```python
from build123d import *

# Parameters (mm, degrees)
ESBO_O1_W                = 12.7
ESBO_O1_H                = 41.5
ESBO_O1_R                = 2.4
RESSALTO_EXTRUS_O1_DEPTH = 3
ESBO_O2_W                = 12.7
ESBO_O2_H                = 3
RESSALTO_EXTRUS_O2_DEPTH = 38.5
ESBO_O3_R                = 2.4
CORTE_EXTRUS_O1_DEPTH    = 41.5
FILETE1_R                = 2


with BuildPart() as part:
    # Esboço1 → Ressalto-extrusão1 (new body)
    with BuildSketch(Plane.XY):
        Rectangle(ESBO_O1_W, ESBO_O1_H)
        with Locations((0, 10.85)):
            Circle(ESBO_O1_R, mode=Mode.SUBTRACT)
        with Locations((0, -8.15)):
            Circle(ESBO_O1_R, mode=Mode.SUBTRACT)
    extrude(amount=RESSALTO_EXTRUS_O1_DEPTH)

    # Esboço2 → Ressalto-extrusão2 (add)
    with BuildSketch(Plane.XY.offset(3)):
        with Locations((0, -19.25)):
            Rectangle(ESBO_O2_W, ESBO_O2_H)
    extrude(amount=RESSALTO_EXTRUS_O2_DEPTH)

    # Esboço3 → Corte-extrusão1 (cut)
    with BuildSketch(Plane(origin=(0, -17.75, 0), x_dir=(1, 0, 0), z_dir=(0, 1, 0))):
        with Locations((0, -12)):
            Circle(ESBO_O3_R)
        with Locations((0, -32)):
            Circle(ESBO_O3_R)
    extrude(amount=-CORTE_EXTRUS_O1_DEPTH, mode=Mode.SUBTRACT)

    # Filete1
    filete1_edges = [part.edges().sort_by_distance(p)[0] for p in [
        (6.35, -19.25, 41.5),
        (-6.35, -19.25, 41.5),
        (-6.35, 20.75, 1.5),
        (6.35, 20.75, 1.5),
    ]]
    fillet(filete1_edges, radius=FILETE1_R)


solid = part.part
```
Geometry: final body of the model. Coordinates: model frame, mm. A direction names the side the tool comes from. Give positions to 0.01 mm unless a question says otherwise; leave off trailing zeros. Write each loop counter-clockwise with the first axis right and the second up, starting at its lowest first coordinate (ties: lowest second). Pieces come first, ordered by that corner, then holes.
1. Draft query along Y for faces 3 (the flat face through (0, -20.75, 20)), 4 (the cylindrical face through (-5.78, -19.23, 40.9)), 5 (the flat face through (0, -17.75, 22)), 6 (the cylindrical face through (-0.52, 8.507, 1.479)). Return one class per face: released by +Y, released by -Y, zero draft, split by the parting line, or undercut.
2. Reachability of faces 1 (the flat face through (0, -19, 41.5)), 2 (the flat face through (0, 2, 3)) from +Z, -Z, +X, -X, +Y, -Y: full face, straight path, thin tool, end or side. Return the list, or none.
3. Section query C-C, the plane z = 32. Return loops of the section in (x, y).
4. Section query A-A, the plane x = 0. Return loops of the section in (y, z), then the cut area to 3 significant figures.
5. Section query D-D, the plane z = 19. Return loops of the section in (x, y), then the cut area to 3 significant figures.
6. Line query: probe 1 along Z at (x, y) = (0, -19); probe 2 along Y at (x, z) = (0, 2); probe 3 along X at (y, z) = (-19, 32). Output: solid intervals per line, ascending.
7. Pin query (flat end, axial travel): P1, Ø6, axis at x = 0, z = 32, coming from the -Y side; P2, Ø4, axis at x = -4, y = -5.5, coming from the +Z side; P3, Ø4, axis at x = 0.5, z = 28.5, coming from the +Y side. Return the tip coordinate at first contact, or that it passes through.
8. Section query B-B, the plane y = -8.15. Return loops of the section in (x, z), then the cut area to 3 significant figures.
Computed:
1. face 3: released by -Y
1. face 4: zero draft
1. face 5: released by +Y
1. face 6: undercut
2. face 1: +Z, +X, -X, +Y, -Y
2. face 2: +Z, +X, -X, +Y
3. outline: (-6.35, -20.75) - (-2.4, -20.75) - (-2.4, -17.75) - (-6.35, -17.75) - close; (2.4, -20.75) - (6.35, -20.75) - (6.35, -17.75) - (2.4, -17.75) - close
4. outline: (-20.75, 0) - (-10.55, 0) - (-10.55, 3) - (-17.75, 3) - (-17.75, 9.6) - (-20.75, 9.6) - close; (-20.75, 14.4) - (-17.75, 14.4) - (-17.75, 29.6) - (-20.75, 29.6) - close; (-20.75, 34.4) - (-17.75, 34.4) - (-17.75, 41.5) - (-20.75, 41.5) - close; (-5.75, 0) - (8.45, 0) - (8.45, 3) - (-5.75, 3) - close; (13.25, 0) - (20.75, 0) - (20.75, 3) - (13.25, 3) - close
4. area: 182 mm2
5. outline: (-6.35, -20.75) - (6.35, -20.75) - (6.35, -17.75) - (-6.35, -17.75) - close
5. area: 38.1 mm2
6. probe 1: z = 0 to 9.6, 14.4 to 29.6, 34.4 to 41.5
6. probe 2: y = -20.75 to -10.55, -5.75 to 8.45, 13.25 to 20.75
6. probe 3: x = -6.35 to -2.4, 2.4 to 6.35
7. P1: stops at y = -20.75
7. P2: stops at z = 3
7. P3: stops at y = -17.75
8. outline: (-6.35, 0) - (-2.4, 0) - (-2.4, 3) - (-6.35, 3) - close; (2.4, 0) - (6.35, 0) - (6.35, 3) - (2.4, 3) - close
8. area: 23.7 mm2
